Geometry check sheet. Reference: the model listing, model coordinates, mm. Round coordinates to 2 decimals unless told otherwise and drop trailing zeros. Loops run counter-clockwise (first coordinate to the right, second up) from the corner with the lowest first, then second, coordinate; pieces in that order, holes last. Notation, with made-up numbers: (28.5, 69.25) - (33.5, 69.25) arc R15 ccw to (33.5, 94.25) - close; hole circle Ø8 at (10.25, -39.5). An arc over 180 degrees is marked (long way). Write item = value, one per line.
```python
from build123d import *

# Parameters (mm, degrees)
F1_DEPTH = 6.35
F2_D     = 5.1054


with BuildPart() as f1:
    # F0 (on Front) → F1 (new body)
    with BuildSketch(Plane.XZ):
        with BuildLine():
            Line((-171.45, -279.4), (171.45, -279.4))
            ThreePointArc((171.45, -279.4), (175.9401280605, -277.5401280605), (177.8, -273.05))
            Line((177.8, -273.05), (177.8, 273.05))
            ThreePointArc((177.8, 273.05), (175.9401280605, 277.5401280605), (171.45, 279.4))
            Line((171.45, 279.4), (-171.45, 279.4))
            ThreePointArc((-171.45, 279.4), (-175.9401280605, 277.5401280605), (-177.8, 273.05))
            Line((-177.8, 273.05), (-177.8, -273.05))
            ThreePointArc((-177.8, -273.05), (-175.9401280605, -277.5401280605), (-171.45, -279.4))
        make_face()
        with BuildLine():
            Line((133.5151, -196.85), (133.5151, -234.95))
            ThreePointArc((133.5151, -234.95), (127, -241.4651), (120.4849, -234.95))
            Line((120.4849, -234.95), (120.4849, -196.85))
            ThreePointArc((120.4849, -196.85), (127, -190.3349), (133.5151, -196.85))
        make_face(mode=Mode.SUBTRACT)
        with BuildLine():
            ThreePointArc((120.4849, 234.95), (127, 241.4651), (133.5151, 234.95))
            Line((133.5151, 234.95), (133.5151, 196.85))
            ThreePointArc((133.5151, 196.85), (127, 190.3349), (120.4849, 196.85))
            Line((120.4849, 196.85), (120.4849, 234.95))
        make_face(mode=Mode.SUBTRACT)
    extrude(amount=F1_DEPTH)

    # F2 (through all)
    with Locations(Plane(origin=(0, 0, 0), x_dir=(1, 0, 0), z_dir=(0, 1, 0))):
        with Locations((139.7, 266.7), (139.7, 133.35), (139.7, 0), (139.7, -133.35), (139.7, -266.7), (-152.4, 266.7), (-152.4, 0), (-152.4, -133.35), (-152.4, -266.7), (-152.4, 133.35)):
            Hole(F2_D / 2)


solid = f1.part
```
(1) Scan lines: L1, parallel to X at y = -1.75, z = 266.7; L2, parallel to Z at x = 139.7, y = -2.5; L3, parallel to Z at x = 140, y = -3. Record each from-to range of solid material in increasing order. Write a range as [from, to].
Answers follow:
L1 = [-177.8, -154.95], [-149.85, 137.15], [142.25, 177.8]
L2 = [-279.4, -269.25], [-264.15, -135.9], [-130.8, -2.55], [2.55, 130.8], [135.9, 264.15], [269.25, 279.4]
L3 = [-279.4, -269.24], [-264.16, -135.89], [-130.81, -2.54], [2.54, 130.81], [135.89, 264.16], [269.24, 279.4]
(2) Section check A-A (z = -224.5). Enter the section's corners in (x, y), then the cut area to 3 significant figures.
Answers follow:
outline = (-177.8, -6.35) - (120.48, -6.35) - (120.48, 0) - (-177.8, 0) - close; (133.52, -6.35) - (177.8, -6.35) - (177.8, 0) - (133.52, 0) - close
area = 2,180 mm²
(3) Gauge pin test, flat end, axial feed: pin 1 (6 mm diameter, centred on x = -152.4, z = -133.35, fed in from -Y). Record the tip position at first contact, or that the pin passes through.
Answers follow:
pin_1 = -6.35
(4) Section check B-B (x = 127). Enter the section's corners in (y, z).
Answers follow:
outline = (-6.35, -279.4) - (0, -279.4) - (0, -241.47) - (-6.35, -241.47) - close; (-6.35, -190.33) - (0, -190.33) - (0, 190.33) - (-6.35, 190.33) - close; (-6.35, 241.47) - (0, 241.47) - (0, 279.4) - (-6.35, 279.4) - close
